Design review of the part shown in the three views and the two pictorial views. Dimensions are in mm from the part's minimum x, y and z. A direction names the side the tool comes from. Round coordinates to 2 decimals unless told otherwise and drop trailing zeros. Write each loop counter-clockwise with the first axis right and the second up, starting at its lowest first coordinate (ties: lowest second). Pieces come first, ordered by that corner, then holes. Notation, with made-up numbers: (83, -28) -> (136, -28) arc R18 cw to (136, 7) -> close; hole circle Ø6 at (-35, 56). An arc over 180 degrees is marked (long way). Return JSON: item names as keys, results as strings. Group by question number.
1. Clearance check with flat-ended pins moving along their axes: P1, Ø5, axis at y = 9, z = 26, coming from the +X side; P2, Ø8, axis at y = 12, z = 10.5, coming from the +X side; P3, Ø6, axis at y = 9.5, z = 20, coming from the -X side. State where each tip first meets the part, or that it passes through.
2. For line 1 along Z through (x, y) = (8.75, 3); line 2 along X through (y, z) = (8.25, 14); line 3 along Y through (x, z) = (7.75, 24.75), list the stretches that pass through material, from the lowest coordinate up. Write a range as from..to.
3. Take a section at D-D, the plane x = 3. Write out the cut boundary in (y, z), then the cut area to 3 significant figures.
4. Take a section at C-C, the plane z = 12. Write out the cut boundary in (x, y), then the cut area to 3 significant figures.
5. Tool access review of the marked faces 3 and 4: name each direction out of +Z, -Z, +X, -X, +Y, -Y from which nothing blocks a thin tool from reaching the whole face with its end or side.
6. Take a section at A-A, the plane x = 7.5. Write out the cut boundary in (y, z).
7. Mouldability with a two-part tool opening along X and no side actions: class the marked faces 1 and 2 as pulls with the +X half, pulls with the -X half, needs draft (parallel to the pull), parting line crosses it, or undercut.
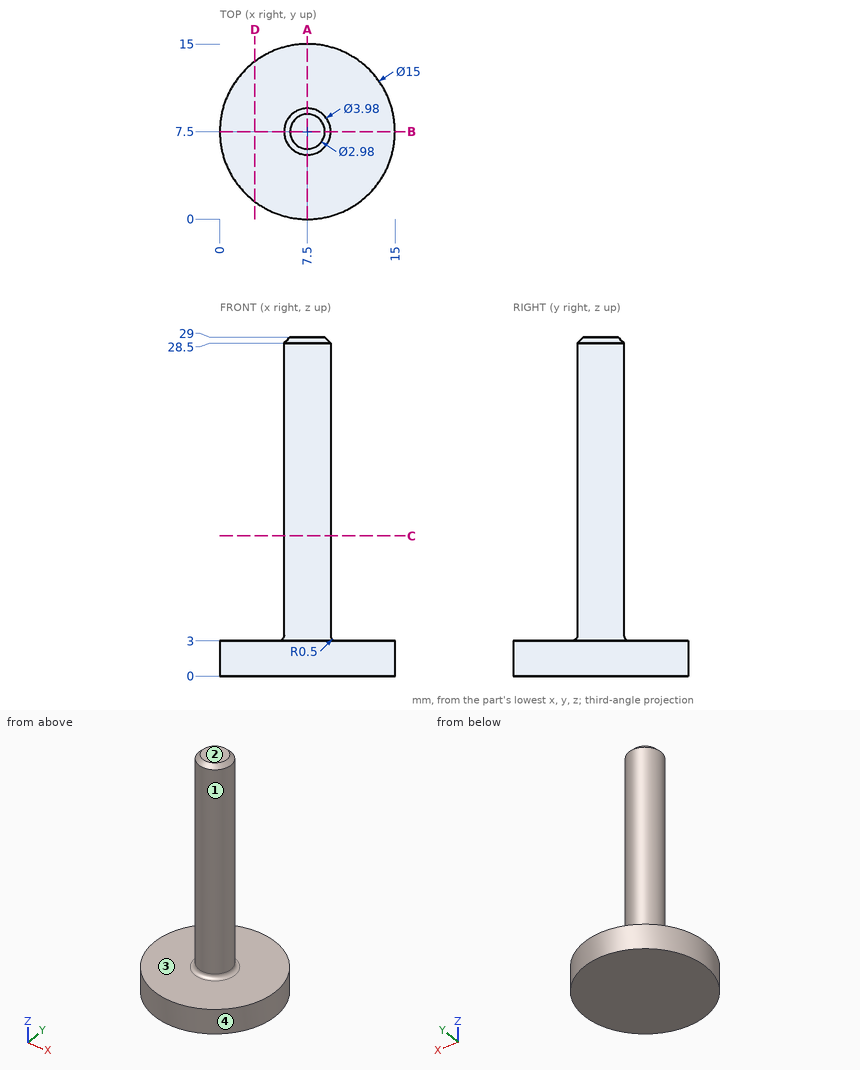
Output:
{
 "1": {"P1": "stops at x = 9.49", "P2": "stops at x = 9.43", "P3": "stops at x = 5.51"},
 "2": {"line 1": "z = 0..3", "line 2": "x = 5.66..9.34", "line 3": "y = 5.53..9.47"},
 "3": {"outline": "(1.5, 0) -> (13.5, 0) -> (13.5, 3) -> (1.5, 3) -> close", "area": "36.0 mm^2"},
 "4": {"outline": "circle Ø3.98 at (7.5, 7.5)", "area": "12.4 mm^2"},
 "5": {"face 3": "+Z", "face 4": "+Z, -Z"},
 "6": {"outline": "(0, 0) -> (15, 0) -> (15, 3) -> (9.99, 3) arc R0.5 cw to (9.49, 3.5) -> (9.49, 28.5) -> (8.99, 29) -> (6.01, 29) -> (5.51, 28.5) -> (5.51, 3.5) arc R0.5 cw to (5.01, 3) -> (0, 3) -> close"},
 "7": {"face 1": "parting line crosses it", "face 2": "needs draft"}
}
